Autodesk Inventor part; units mm, degrees
ref_plane "YZ Plane" through (0, 0, 0) normal (1, 0, 0) x (0, 1, 0)
ref_plane "XZ Plane" through (0, 0, 0) normal (0, 1, 0) x (-1, 0, 0)
ref_plane "XY Plane" through (0, 0, 0) normal (0, 0, 1) x (1, 0, 0)
sketch "Sketch1" plane through (0, 0, 0) normal (0, 0, 1) x (1, 0, 0)
  circle A0 centre (0, 0) radius 35
  dimension "d4" = 70
extrude "Extrusion1" add sketch "Sketch1" along normal blind 10
sketch "Sketch2" plane through (0, 0, 0) normal (0, 0, -1) x (-1, 0, 0)
  circle A0 centre (19.9717, 6.4907) radius 2.5
  circle A1 centre (6.7998, -20.9228) radius 2.5
  circle A2 centre (-19.9717, -6.4907) radius 2.5
  circle A3 centre (-6.7998, 20.9228) radius 2.5
sketch3d "3D Sketch1"
hole "Hole2" at (0, 0, 0) direction (0, 0, 1) diameter 10 end through all
hole "Hole5" at (6.7998, 20.9228, 0) at (19.9717, -6.4907, 0) at (-6.7998, -20.9228, 0) direction (0, 0, 1) diameter 5 end through all
properties part number "Plate"
Input: part model. Units: mm. Frame: model coordinates. Coordinates: 2 decimals unless noted, no trailing zeros. Order: outer loops, then holes, each group sorted by start corner. A loop starts at its lowest first (then second) coordinate and runs counter-clockwise, first axis right, second up. Notation, with made-up numbers: M 34.5,58 L 61.5,58 A26 cw 61.5,86 Z; hole C -19.75,40.5 d4. An arc over 180 degrees is marked long. Write item = value, one per line. Start each with the question number.
(1) Section C-C on z = 3. Output: boundary loops of the cut face in (x, y), and give its area (3 significant figures).
(2) First-contact query: P1, Ø1.5, axis at x = -16.5, z = 4.5, coming from the -Y side; P2, Ø1, axis at x = 24.5, z = 6, coming from the -Y side; P3, Ø2, axis at x = 10.5, z = 7.5, coming from the -Y side; P4, Ø6, axis at x = 0, y = 0, coming from the +Z side. Flat tips, straight axial feed; report the tip coordinate or a pass-through.
(3) Section D-D on x = 15. Output: boundary loops of the cut face in (y, z).
(4) Pull-direction query (X, two-part tool) for faces 1 (the cylindrical face through (4.88, -1.08, 5.07)), 2 (the flat face through (7, 0, 0)), 3 (the cylindrical face through (-28, 21, 5)), 4 (the cylindrical face through (22.19, -5.34, 5.07)); classes: released by +X, released by -X, zero draft, split by the parting line, or undercut.
(5) Line query: line 1 along Y through (x, z) = (0, 5); line 2 along X through (y, z) = (2, 3.25); line 3 along Y through (x, z) = (7.5, 8.5). Output: solid intervals per line, ascending. Write a range as [from, to].
(6) Section A-A on x = 0. Output: boundary loops of the cut face in (y, z).
Result set:
q1.outline = C 0,0 d70; hole C -6.8,-20.92 d5; hole C 0,0 d10; hole C 6.8,20.92 d5; hole C 19.97,-6.49 d5
q1.area = 3,710 mm²
q2.P1 = -31.26
q2.P2 = -25.48
q2.P3 = -33.69
q2.P4 = through
q3.outline = M -31.62,0 L 31.62,0 L 31.62,10 L -31.62,10 Z
q4.face_1 = undercut
q4.face_2 = zero draft
q4.face_3 = split by the parting line
q4.face_4 = undercut
q5.line_1 = [-35, -5], [5, 35]
q5.line_2 = [-34.94, -4.58], [4.58, 34.94]
q5.line_3 = [-34.19, 18.52], [23.32, 34.19]
q6.outline = M -35,0 L -5,0 L -5,10 L -35,10 Z; M 5,0 L 35,0 L 35,10 L 5,10 Z
